Model file for the job. Use its own axes, mm. A direction names the side the tool comes from. Round coordinates to 2 decimals unless told otherwise and drop trailing zeros. Loops run counter-clockwise (first coordinate to the right, second up) from the corner with the lowest first, then second, coordinate; pieces in that order, holes last. Notation, with made-up numbers: M 65.5,72 L 94.5,72 A16 ccw 94.5,88 Z; hole C 72.25,30 d6. An arc over 180 degrees is marked long. Use a Markdown table: item, result. Add a question column.
Q1. Tool access for faces 1 (the face through (25, 30, -29)), 2 (the face through (0, 30, 30)), 3 (the face through (-27.5, 28, 0)): list every direction of +Z, -Z, +X, -X, +Y, -Y with a clear straight run to the whole face (end or side of a thin tool).
Q2. Cut at B-B (z = 10.5). Give the cut face in (x, y).
Q3. Cut at A-A (x = 13.5). Give the cut face in (y, z), plus the area to 3 significant figures.
Q4. Pin check, flat tips, straight feed: pin 1 (5 mm diameter, centred on x = 9.5, z = 13, fed in from -Y); pin 2 (3 mm diameter, centred on x = 7, y = 29, fed in from -Z). Stop position of each tip, or through.
Q5. Mould opens along X. For faces 4 (the face through (0, 57.5, 0)), 5 (the face through (30, 30, 0)), 6 (the face through (-2, 0, 29)) say: +X half, -X half, draft (parallel to the pull), parting line (faces both ways), or undercut.
Q6. Probe line 1 (X direction, y = 38, z = -1); line 2 (Z direction, x = 20, y = 39). List the from-to ranges inside material, lowest first. Write a range as from..to.
Q7. Cut at C-C (y = 18.5). Give the cut face in (x, z).
from build123d import *

# Parameters (mm, degrees)
SKETCH1_W           = 60
SKETCH1_H           = 60
BOSS_EXTRUDE1_DEPTH = 60
SKETCH2_W           = 55
SKETCH2_H           = 55
BOSS_EXTRUDE2_DEPTH = 57.5
SKETCH2_2_W         = 55
SKETCH2_2_H         = 55
CUT_EXTRUDE1_DEPTH  = 57.5
SKETCH5_W           = 50
SKETCH5_H           = 50
CUT_EXTRUDE2_DEPTH  = 20
SKETCH6_W           = 30
SKETCH6_H           = 3.5
CUT_EXTRUDE3_DEPTH  = 20
SKETCH7_R           = 0.5
CUT_EXTRUDE4_DEPTH  = 3.3


with BuildPart() as part:
    # Sketch1 → Boss-Extrude1 (new body)
    with BuildSketch(Plane(origin=(0, 0, 0), x_dir=(1, 0, 0), z_dir=(0, 1, 0))):
        Rectangle(SKETCH1_W, SKETCH1_H)
    extrude(amount=BOSS_EXTRUDE1_DEPTH)

    # Sketch2 → Boss-Extrude2 (add)
    with BuildSketch(Plane.XZ):
        Rectangle(SKETCH2_W, SKETCH2_H)
    extrude(amount=-BOSS_EXTRUDE2_DEPTH)

    # Sketch2<2> → Cut-Extrude1 (cut)
    with BuildSketch(Plane.XZ):
        Rectangle(SKETCH2_2_W, SKETCH2_2_H)
    extrude(amount=-CUT_EXTRUDE1_DEPTH, mode=Mode.SUBTRACT)

    # Sketch5 → Cut-Extrude2 (cut)
    with BuildSketch(Plane(origin=(0, 0, -30), x_dir=(-1, 0, 0), z_dir=(0, 0, -1))):
        with Locations((0, 30)):
            Rectangle(SKETCH5_W, SKETCH5_H)
    extrude(amount=-CUT_EXTRUDE2_DEPTH, mode=Mode.SUBTRACT)

    # Sketch6 → Cut-Extrude3 (cut)
    with BuildSketch(Plane(origin=(0, 0, -30), x_dir=(-1, 0, 0), z_dir=(0, 0, -1))):
        with Locations((0, 3)):
            Rectangle(SKETCH6_W, SKETCH6_H)
    extrude(amount=-CUT_EXTRUDE3_DEPTH, mode=Mode.SUBTRACT)

    # Sketch7 → Cut-Extrude4 (cut)
    with BuildSketch(Plane(origin=(0, 0, -30), x_dir=(-1, 0, 0), z_dir=(0, 0, -1))):
        with Locations((10, 0.6)):
            Circle(SKETCH7_R)
    cut_extrude4 = extrude(amount=-CUT_EXTRUDE4_DEPTH, mode=Mode.SUBTRACT)

    # Mirror1: Cut-Extrude4 across plane
    add(cut_extrude4.mirror(Plane.ZY), mode=Mode.SUBTRACT)


solid = part.part
Checked values:
| question | item | result |
|---|---|---|
| 1 | face 1 | -Z |
| 1 | face 2 | +Z, +X, -X, +Y, -Y |
| 1 | face 3 | -Y |
| 2 | outline | M -30,0 L -27.5,0 L -27.5,57.5 L 27.5,57.5 L 27.5,0 L 30,0 L 30,60 L -30,60 Z |
| 3 | outline | M 0,-30 L 1.25,-30 L 1.25,-27.5 L 0,-27.5 Z; M 0,27.5 L 57.5,27.5 L 57.5,-27.5 L 55,-27.5 L 55,-30 L 60,-30 L 60,30 L 0,30 Z; M 4.75,-30 L 5,-30 L 5,-27.5 L 4.75,-27.5 Z |
| 3 | area | 304 mm^2 |
| 4 | pin 1 | stops at y = 57.5 |
| 4 | pin 2 | stops at z = 27.5 |
| 5 | face 4 | undercut |
| 5 | face 5 | +X half |
| 5 | face 6 | draft |
| 6 | line 1 | x = -30..-27.5, 27.5..30 |
| 6 | line 2 | z = 27.5..30 |
| 7 | outline | M -30,-30 L -25,-30 L -25,-27.5 L -27.5,-27.5 L -27.5,27.5 L 27.5,27.5 L 27.5,-27.5 L 25,-27.5 L 25,-30 L 30,-30 L 30,30 L -30,30 Z |
